from build123d import *

# Parameters (mm, degrees)
SKETCH2_W           = 260.35
SKETCH2_H           = 20.32
SKETCH2_R           = 3.1877
BOSS_EXTRUDE1_DEPTH = 6.35
SKETCH3_W           = 19.5072
SKETCH3_H           = 5.9436
CUT_EXTRUDE1_DEPTH  = 261.625537122
SKETCH4_W           = 25.4
SKETCH4_H           = 5.3975
CUT_EXTRUDE2_DEPTH  = 131.725203098


with BuildPart() as part:
    # Sketch2 → Boss-Extrude1 (new body)
    with BuildSketch(Plane(origin=(0, 0, 0), x_dir=(1, 0, 0), z_dir=(0, 1, 0))):
        Rectangle(SKETCH2_W, SKETCH2_H)
        with Locations(Location((-117.475, 0, 0), (0, 0, 270))):
            Circle(SKETCH2_R, mode=Mode.SUBTRACT)
        with Locations(Location((117.475, 0, 0), (0, 0, 270))):
            Circle(SKETCH2_R, mode=Mode.SUBTRACT)
    extrude(amount=-BOSS_EXTRUDE1_DEPTH)

    # Sketch3 → Cut-Extrude1 (cut, through all)
    with BuildSketch(Plane(origin=(130.175, 0, 0), x_dir=(0, 0, -1), z_dir=(1, 0, 0))):
        with Locations((0, -3.3782)):
            Rectangle(SKETCH3_W, SKETCH3_H)
    extrude(amount=-CUT_EXTRUDE1_DEPTH, mode=Mode.SUBTRACT)

    # Sketch4 → Cut-Extrude2 (cut, through all)
    with BuildSketch(Plane(origin=(0, 0, 0), x_dir=(1, 0, 0), z_dir=(0, 1, 0))):
        with Locations((-117.475, 7.46125)):
            Rectangle(SKETCH4_W, SKETCH4_H)
        with Locations((-117.475, -7.46125)):
            Rectangle(SKETCH4_W, SKETCH4_H)
        with Locations((117.475, 7.46125)):
            Rectangle(SKETCH4_W, SKETCH4_H)
        with Locations((117.475, -7.46125)):
            Rectangle(SKETCH4_W, SKETCH4_H)
    extrude(amount=-CUT_EXTRUDE2_DEPTH, mode=Mode.SUBTRACT)


solid = part.part
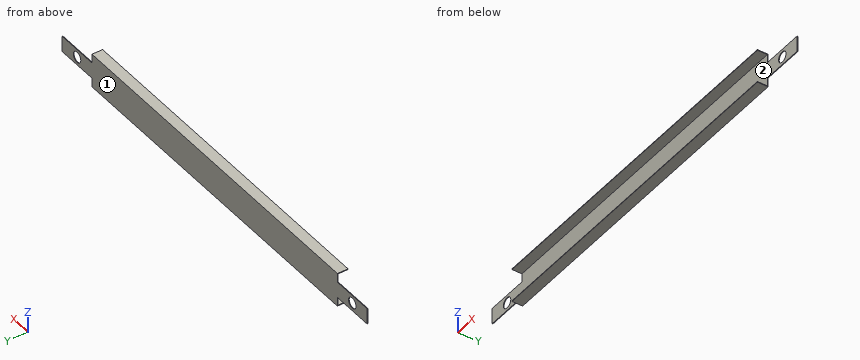
Part model, mm, in its own coordinate system. Face numbers are marked on the shaded views. Coordinates: 2 decimals unless noted, no trailing zeros. Order: outer loops, then holes, each group sorted by start corner. A loop starts at its lowest first (then second) coordinate and runs counter-clockwise, first axis right, second up. Notation, with made-up numbers: M -33.5,-3.5 L -15.5,-3.5 A34 cw -15.5,27.5 Z; hole C 13,-10 d8. An arc over 180 degrees is marked long. Use a Markdown table: item, result.
(1) Cut at B-B on y = -3. Write the cut outline in (x, z) (3 decimals), then the cut area to 3 significant figures.
A:
| item | result |
|---|---|
| outline | M -104.775,-10.16 L 104.775,-10.16 L 104.775,-9.754 L -104.775,-9.754 Z; M -104.775,9.754 L 104.775,9.754 L 104.775,10.16 L -104.775,10.16 Z |
| area | 170 mm^2 |
(2) Cut at A-A on z = 0. Write the cut outline in (x, y) (3 decimals).
A:
| item | result |
|---|---|
| outline | M -130.175,-0.406 L -120.663,-0.406 L -120.663,0 L -130.175,0 Z; M -114.287,-0.406 L 114.287,-0.406 L 114.287,0 L -114.287,0 Z; M 120.663,-0.406 L 130.175,-0.406 L 130.175,0 L 120.663,0 Z |
(3) Probe L1, parallel to Z at x = -38, y = -4.5; L2, parallel to X at y = -0.3, z = 0 (3 decimals); L3, parallel to Y at x = -58.5, z = -4. List the from-to ranges inside material, lowest first.
A:
| item | result |
|---|---|
| L1 | z = -10.16 to -9.75, 9.75 to 10.16 |
| L2 | x = -130.175 to -120.663, -114.287 to 114.287, 120.663 to 130.175 |
| L3 | y = -0.41 to 0 |
(4) Pull direction Z, two halves, no side cores. Call the marked faces 1 and 2: released by +Z, released by -Z, zero draft, split by the parting line, or undercut.
A:
| item | result |
|---|---|
| face 1 | zero draft |
| face 2 | undercut |
(5) Cut at C-C on x = -75. Write the cut outline in (y, z).
A:
| item | result |
|---|---|
| outline | M -6.35,-10.16 L 0,-10.16 L 0,10.16 L -6.35,10.16 L -6.35,9.75 L -0.41,9.75 L -0.41,-9.75 L -6.35,-9.75 Z |
(6) Flat gauge pins, fed straight in: pin 1 (5 mm diameter, centred on x = -117.475, z = 0, fed in from +Y); pin 2 (12 mm diameter, centred on x = 61.5, z = 2, fed in from -Y). Where does each tip first touch, or does it go through?
A:
| item | result |
|---|---|
| pin 1 | passes through |
| pin 2 | stops at y = -0.41 |
